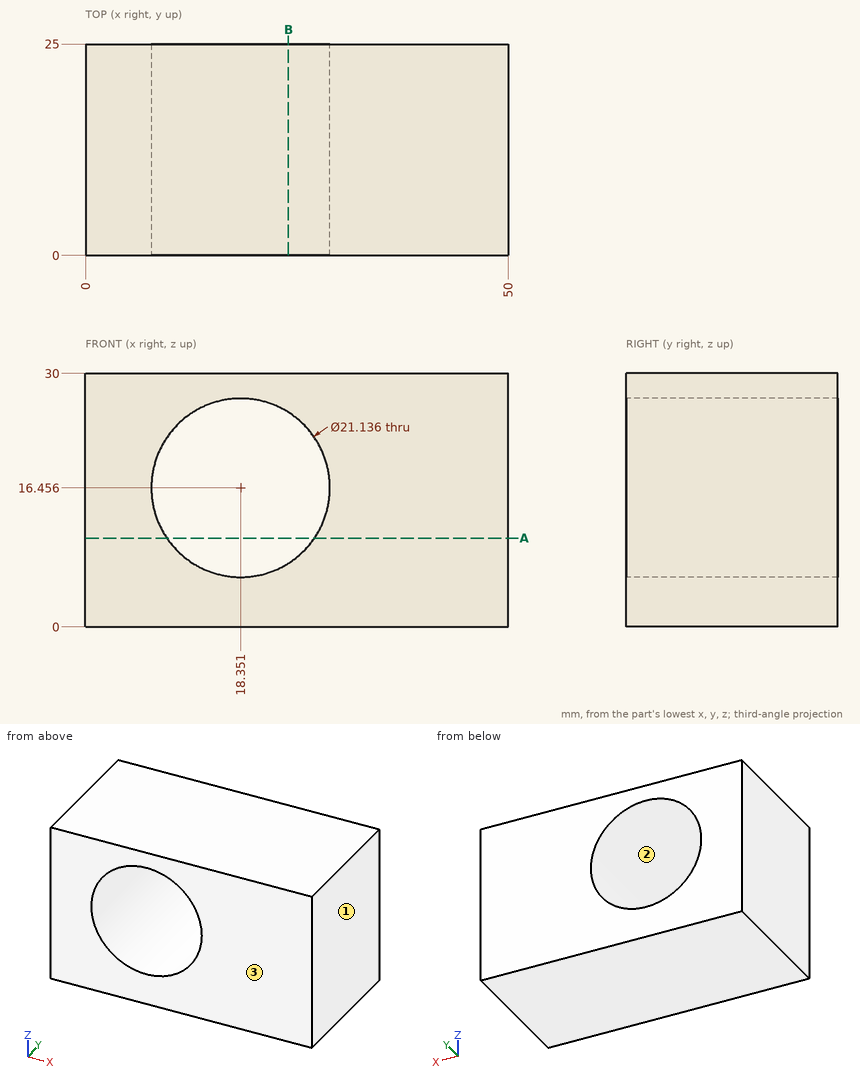
Check sheet for the drawn part. Datum: minimum x, y, z corner. Units: mm. Give positions to 0.01 mm unless a question says otherwise; leave off trailing zeros. Order: outer loops, then holes, each group sorted by start corner. A loop starts at its lowest first (then second) coordinate and runs counter-clockwise, first axis right, second up. Notation, with made-up numbers: (-32.75, 73.5) -> (-11.75, 73.5) arc R25 ccw to (-11.75, 88.5) -> close; hole circle Ø8 at (35.25, -0.5). An arc over 180 degrees is marked (long way). Return JSON: item names as keys, results as strings.
1. Material ranges on probe 1 along Z at (x, y) = (23, 15.75) (1 decimal); probe 2 along X at (y, z) = (18.25, 14.5) (1 decimal); probe 3 along X at (y, z) = (14.25, 17) (1 decimal), recorded low to high. Write a range as [from, to].
From the geometry:
{"probe 1": "[0, 7], [25.9, 30]", "probe 2": "[0, 8], [28.7, 50]", "probe 3": "[0, 7.8], [28.9, 50]"}
2. Cross-section at A-A, the plane z = 10.5. Record the cut outline in (x, y).
From the geometry:
{"outline": "(0, 0) -> (9.62, 0) -> (9.62, 25) -> (0, 25) -> close; (27.08, 0) -> (50, 0) -> (50, 25) -> (27.08, 25) -> close"}
3. Cross-section at B-B, the plane x = 24. Record the cut outline in (y, z) (1 decimal).
From the geometry:
{"outline": "(0, 0) -> (25, 0) -> (25, 7.5) -> (0, 7.5) -> close; (0, 25.4) -> (25, 25.4) -> (25, 30) -> (0, 30) -> close"}
4. Mould release check, pull along X, two halves, no side actions. Record for the marked faces 1, 2 and 3: +X half, -X half, draft (parallel to the pull), parting line (faces both ways), or undercut.
From the geometry:
{"face 1": "+X half", "face 2": "undercut", "face 3": "draft"}
